from build123d import *

# Parameters (mm, degrees)
F1_DEPTH = 5
F0_R     = 2.5
F2_DEPTH = 10
F3_ANGLE = 180
F4_DEPTH = 45


# Not quite as in the source:
# - a feature names something its author has since deleted; it is built from what else it names


with BuildPart() as f1:
    # F0 (on Front) → F1 (new body)
    with BuildSketch(Plane.XZ):
        with BuildLine():
            Line((52.5, 64.0237609195), (-52.5, 64.0237609195))
            Line((-52.5, 64.0237609195), (-161.030379156, 126.1777225507))
            ThreePointArc((-161.030379156, 126.1777225507), (-157.3485201139, 122.5151665755), (-156, 117.5))
            ThreePointArc((-156, 117.5), (-160.9848334245, 108.8485201139), (-170.969620844, 108.8222774493))
            Line((-170.969620844, 108.8222774493), (-72.6222594518, 52.5))
            Line((-72.6222594518, 52.5), (-72.6222594518, -52.5))
            Line((-72.6222594518, -52.5), (-170.969620844, -108.8222774493))
            ThreePointArc((-170.969620844, -108.8222774493), (-160.9848334245, -108.8485201139), (-156, -117.5))
            ThreePointArc((-156, -117.5), (-157.3485201139, -122.5151665755), (-161.030379156, -126.1777225507))
            Line((-161.030379156, -126.1777225507), (-52.5, -64.0237609195))
            Line((-52.5, -64.0237609195), (52.5, -64.0237609195))
            Line((52.5, -64.0237609195), (161.030379156, -126.1777225507))
            ThreePointArc((161.030379156, -126.1777225507), (157.3222774493, -112.530379156), (170.969620844, -108.8222774493))
            Line((170.969620844, -108.8222774493), (72.6222594518, -52.5))
            Line((72.6222594518, -52.5), (72.6222594518, 52.5))
            Line((72.6222594518, 52.5), (170.969620844, 108.8222774493))
            ThreePointArc((170.969620844, 108.8222774493), (157.3222774493, 112.530379156), (161.030379156, 126.1777225507))
            Line((161.030379156, 126.1777225507), (52.5, 64.0237609195))
        make_face()
        with BuildLine():
            Line((45, 0), (3.75, 0))
            ThreePointArc((3.75, 0), (0, -3.75), (-3.75, 0))
            Line((-3.75, 0), (-45, 0))
            ThreePointArc((-45, 0), (0, 45), (45, 0))
        make_face(mode=Mode.SUBTRACT)
        with BuildLine():
            ThreePointArc((-3.75, 0), (0, 3.75), (3.75, 0))
            Line((3.75, 0), (45, 0))
            ThreePointArc((45, 0), (0, 45), (-45, 0))
            Line((-45, 0), (-3.75, 0))
        make_face()
    extrude(amount=F1_DEPTH)

    # F0 (on Front) → F2 (join)
    with BuildSketch(Plane.XZ):
        with BuildLine():
            ThreePointArc((-156, 117.5), (-157.3485201139, 122.5151665755), (-161.030379156, 126.1777225507))
            ThreePointArc((-161.030379156, 126.1777225507), (-174.6777225507, 122.469620844), (-170.969620844, 108.8222774493))
            ThreePointArc((-170.969620844, 108.8222774493), (-160.9848334245, 108.8485201139), (-156, 117.5))
        make_face()
        with Locations((-166, 117.5)):
            Circle(F0_R, mode=Mode.SUBTRACT)
        with BuildLine():
            ThreePointArc((176, -117.5), (174.6514798861, -112.4848334245), (170.969620844, -108.8222774493))
            ThreePointArc((170.969620844, -108.8222774493), (157.3222774493, -112.530379156), (161.030379156, -126.1777225507))
            ThreePointArc((161.030379156, -126.1777225507), (171.0151665755, -126.1514798861), (176, -117.5))
        make_face()
        with Locations((166, -117.5)):
            Circle(F0_R, mode=Mode.SUBTRACT)
        with BuildLine():
            ThreePointArc((176, 117.5), (171.0151665755, 126.1514798861), (161.030379156, 126.1777225507))
            ThreePointArc((161.030379156, 126.1777225507), (157.3222774493, 112.530379156), (170.969620844, 108.8222774493))
            ThreePointArc((170.969620844, 108.8222774493), (174.6514798861, 112.4848334245), (176, 117.5))
        make_face()
        with Locations((166, 117.5)):
            Circle(F0_R, mode=Mode.SUBTRACT)
        with BuildLine():
            ThreePointArc((-156, -117.5), (-160.9848334245, -108.8485201139), (-170.969620844, -108.8222774493))
            ThreePointArc((-170.969620844, -108.8222774493), (-174.6777225507, -122.469620844), (-161.030379156, -126.1777225507))
            ThreePointArc((-161.030379156, -126.1777225507), (-157.3485201139, -122.5151665755), (-156, -117.5))
        make_face()
        with Locations((-166, -117.5)):
            Circle(F0_R, mode=Mode.SUBTRACT)
    extrude(amount=F2_DEPTH)

    # F0 (on Front) → F3 (revolve)
    with BuildSketch(Plane.XZ):
        with BuildLine():
            ThreePointArc((-3.75, 0), (0, 3.75), (3.75, 0))
            Line((3.75, 0), (45, 0))
            ThreePointArc((45, 0), (0, 45), (-45, 0))
            Line((-45, 0), (-3.75, 0))
        make_face()
    revolve(axis=Axis((0, 0, 0), (-1, 0, 0)), revolution_arc=F3_ANGLE)

    # F0 (on Front) → F4 (cut)
    with BuildSketch(Plane.XZ):
        with BuildLine():
            ThreePointArc((-3.75, 0), (0, -3.75), (3.75, 0))
            Line((3.75, 0), (-3.75, 0))
        make_face()
        with BuildLine():
            Line((-3.75, 0), (3.75, 0))
            ThreePointArc((3.75, 0), (0, 3.75), (-3.75, 0))
        make_face()
    extrude(amount=-F4_DEPTH, mode=Mode.SUBTRACT)


solid = f1.part
Could you check a few things on this model? Use its own coordinates, in mm. A direction names the side the tool comes from. Coordinates: 2 decimals unless noted, no trailing zeros. Order: outer loops, then holes, each group sorted by start corner. A loop starts at its lowest first (then second) coordinate and runs counter-clockwise, first axis right, second up. Notation, with made-up numbers: (-1.75, -3) - (27.25, -3) arc R25 cw to (27.25, 16) - close; hole circle Ø5 at (48.5, 29). An arc over 180 degrees is marked (long way). Answer in a Markdown table with one row per item. Add a question column.
(1) If we section it at D-D, the plane y = 17.5: Please give me the cut outline in (x, z).
(2) If we mould it in two halves opening along Z, with no side actions, what happens to faces 5 (the face through (107.525, -2.465, 95.536)), 6 (the face through (106.01, -2.46, -94.67)), 7 (the face through (-164, -10, -120)), 8 (the face through (-121.11, -2.46, -80.27))? For each: released by +Z, released by -Z, zero draft, split by the parting line, or undercut.
(3) On a 3-axis mill with a long thin cutter (end or side, diameter ignored), from which of +Z, -Z, +X, -X, +Y, -Y can I reach the whole of each face in a straight line? I mean faces 1 (the face through (121.11, -2.46, 80.27)), 2 (the face through (-106.01, -2.46, 94.67)), 3 (the face through (-122.484, -2.465, 81.055)), 4 (the face through (-107.525, -2.465, -95.536)). Say none if no direction works.
(4) If we section it at B-B, the plane x = -128.5: Please give me the cut outline in (y, z), then the cut area to 3 significant figures.
(5) If we section it at A-A, the plane z = 0: Please give me the cut outline in (x, y).
(6) If we section it at C-C, the plane z = -92.5: Please give me the cut outline in (x, y), then the cut area to 3 significant figures.
(7) Will these pins go through, and if not, where does the flat tip stop? pin 1 (2.5 mm diameter, centred on x = -0.5, y = -3.5, fed in from -Z); pin 2 (2.5 mm diameter, centred on y = -2, z = 1.5, fed in from -X); pin 3 (4.5 mm diameter, centred on x = 0, z = 0, fed in from +Y); pin 4 (5.5 mm diameter, centred on y = -1.5, z = -14, fed in from +X).
(8) I need wall thicknesses on L1, parallel to Z at x = -166, y = -7.75; L2, parallel to X at y = -6, z = 117; L3, parallel to Z at x = -166, y = -3.5. Which ranges of each line are inside material? Lowest first, please.
Results are:
| question | item | result |
|---|---|---|
| 1 | outline | circle Ø82.92 at (0, 0); hole circle Ø7.5 at (0, 0) |
| 2 | face 5 | released by +Z |
| 2 | face 6 | released by -Z |
| 2 | face 7 | zero draft |
| 2 | face 8 | undercut |
| 3 | face 1 | +X, +Y, -Y |
| 3 | face 2 | +Z, +Y, -Y |
| 3 | face 3 | -X, +Y, -Y |
| 3 | face 4 | -Z, +Y, -Y |
| 4 | outline | (-5, -107.55) - (0, -107.55) - (0, -84.5) - (-5, -84.5) - close; (-5, 84.5) - (0, 84.5) - (0, 107.55) - (-5, 107.55) - close |
| 4 | area | 230 mm2 |
| 5 | outline | (-72.62, -5) - (-3.75, -5) - (-3.75, 44.84) arc R45 ccw to (-45, 0) - (-72.62, 0) - close; (3.75, -5) - (72.62, -5) - (72.62, 0) - (45, 0) arc R45 ccw to (3.75, 44.84) - close |
| 6 | outline | (-142.47, -5) - (-102.22, -5) - (-102.22, 0) - (-142.47, 0) - close; (102.22, -5) - (142.47, -5) - (142.47, 0) - (102.22, 0) - close |
| 6 | area | 402 mm2 |
| 7 | pin 1 | stops at z = -64.02 |
| 7 | pin 2 | stops at x = -72.62 |
| 7 | pin 3 | passes through |
| 7 | pin 4 | stops at x = 72.62 |
| 8 | L1 | z = -127.5 to -120, -115 to -107.5, 107.5 to 115, 120 to 127.5 |
| 8 | L2 | x = -175.99 to -168.45, -163.55 to -156.01, 156.01 to 163.55, 168.45 to 175.99 |
| 8 | L3 | z = -127.5 to -120, -115 to -105.98, 105.98 to 115, 120 to 127.5 |
